from build123d import *

# Parameters (mm, degrees)
SKETCH_1_W          = 54
SKETCH_1_H          = 54
EXTRUDE_1_DEPTH     = 24
FILLET_1_R          = 2
FILLET_2_R          = 2
FILLET_3_R          = 2
FILLET_4_R          = 2
CUT_EXTRUDE_1_DEPTH = 20
SKETCH_9_R          = 2.5
SKETCH_9_R_2        = 0.75
EXTRUDE_4_DEPTH     = 6.4


with BuildPart() as part:
    # Sketch 1 → Extrude 1 (new body)
    with BuildSketch(Plane(origin=(0, 0, 0), x_dir=(1, 0, 0), z_dir=(0, 1, 0))):
        Rectangle(SKETCH_1_W, SKETCH_1_H)
    extrude(amount=EXTRUDE_1_DEPTH)

    # Fillet 1
    fillet_1_edges = [part.edges().sort_by_distance(p)[0] for p in [
        (-27, 12, 27),
    ]]
    fillet(fillet_1_edges, radius=FILLET_1_R)

    # Fillet 2
    fillet_2_edges = [part.edges().sort_by_distance(p)[0] for p in [
        (-27, 12, -27),
    ]]
    fillet(fillet_2_edges, radius=FILLET_2_R)

    # Fillet 3
    fillet_3_edges = [part.edges().sort_by_distance(p)[0] for p in [
        (27, 12, 27),
    ]]
    fillet(fillet_3_edges, radius=FILLET_3_R)

    # Fillet 4
    fillet_4_edges = [part.edges().sort_by_distance(p)[0] for p in [
        (27, 12, -27),
    ]]
    fillet(fillet_4_edges, radius=FILLET_4_R)

    # Sketch 6 → Cut-Extrude 1 (cut)
    with BuildSketch(Plane.XZ):
        with BuildLine():
            Line((-25.5, 25), (-25.5, -25))
            ThreePointArc((-25.5, -25), (-25.353553391, -25.353553391), (-25, -25.5))
            Line((-25, -25.5), (25, -25.5))
            ThreePointArc((25, -25.5), (25.353553391, -25.353553391), (25.5, -25))
            Line((25.5, -25), (25.5, 25))
            ThreePointArc((25.5, 25), (25.353553391, 25.353553391), (25, 25.5))
            Line((25, 25.5), (-25, 25.5))
            ThreePointArc((-25, 25.5), (-25.353553391, 25.353553391), (-25.5, 25))
        make_face()
    extrude(amount=-CUT_EXTRUDE_1_DEPTH, mode=Mode.SUBTRACT)

    # Sketch 9 → Extrude 4 (add)
    # profile 1 of 4: a face of its own
    with BuildSketch(Plane.XZ.offset(-20)):
        with Locations(Location((22.15, -22.5, 0), (0, 0, 270))):
            Circle(SKETCH_9_R)
        with Locations(Location((22.15, -22.5, 0), (0, 0, 270))):
            Circle(SKETCH_9_R_2, mode=Mode.SUBTRACT)
    # profile 2 of 4: a face of its own
    with BuildSketch(Plane.XZ.offset(-20)):
        with Locations(Location((-22.15, -22.5, 0), (0, 0, 270))):
            Circle(SKETCH_9_R)
        with Locations(Location((-22.15, -22.5, 0), (0, 0, 270))):
            Circle(SKETCH_9_R_2, mode=Mode.SUBTRACT)
    # profile 3 of 4: a face of its own
    with BuildSketch(Plane.XZ.offset(-20)):
        with Locations(Location((22.15, 11.8, 0), (0, 0, 270))):
            Circle(SKETCH_9_R)
        with Locations(Location((22.15, 11.8, 0), (0, 0, 270))):
            Circle(SKETCH_9_R_2, mode=Mode.SUBTRACT)
    # profile 4 of 4: a face of its own
    with BuildSketch(Plane.XZ.offset(-20)):
        with Locations(Location((-22.15, 11.8, 0), (0, 0, 270))):
            Circle(SKETCH_9_R)
        with Locations(Location((-22.15, 11.8, 0), (0, 0, 270))):
            Circle(SKETCH_9_R_2, mode=Mode.SUBTRACT)
    extrude(amount=EXTRUDE_4_DEPTH)


solid = part.part
Build history of the part. All positions in model axes, mm. A direction names the side the tool comes from. Round coordinates to 2 decimals unless told otherwise and drop trailing zeros. Loops run counter-clockwise (first coordinate to the right, second up) from the corner with the lowest first, then second, coordinate; pieces in that order, holes last. Notation, with made-up numbers: (-17, 27) -> (-2, 27) arc R29 cw to (-2, 59) -> close; hole circle Ø3 at (10, 55). An arc over 180 degrees is marked (long way). Answer in a Markdown table with one row per item.
Item 1: Pin check, flat tips, straight feed: pin 1 (0.8 mm diameter, centred on x = -22.5, z = -23, fed in from -Y); pin 2 (8 mm diameter, centred on x = -11, z = -0.5, fed in from -Y). Stop position of each tip, or through.
Answers below:
| item | result |
|---|---|
| pin 1 | stops at y = 13.6 |
| pin 2 | stops at y = 20 |
Item 2: Saw through at D-D (x = -15.5). Write the cut outline in (y, z), and give its area (3 significant figures).
Answers below:
| item | result |
|---|---|
| outline | (0, -27) -> (24, -27) -> (24, 27) -> (0, 27) -> (0, 25.5) -> (20, 25.5) -> (20, -25.5) -> (0, -25.5) -> close |
| area | 276 mm² |
Item 3: Which spindle directions (+Z, -Z, +X, -X, +Y, -Y) get a long thin tool onto all of the face, cutting with end or side? Do faces 4 (the cylindrical face through (22.18, 16.84, -21.75)), 5 (the flat face through (-2, 0, 26)). Say none if no direction does.
Answers below:
| item | result |
|---|---|
| face 4 | -Y |
| face 5 | +Z, -Z, +X, -X, -Y |
Item 4: Saw through at B-B (z = -22.5). Write the cut outline in (x, y), and give its area (3 significant figures).
Answers below:
| item | result |
|---|---|
| outline | (-27, 0) -> (-25.5, 0) -> (-25.5, 20) -> (-24.65, 20) -> (-24.65, 13.6) -> (-22.9, 13.6) -> (-22.9, 20) -> (-21.4, 20) -> (-21.4, 13.6) -> (-19.65, 13.6) -> (-19.65, 20) -> (19.65, 20) -> (19.65, 13.6) -> (21.4, 13.6) -> (21.4, 20) -> (22.9, 20) -> (22.9, 13.6) -> (24.65, 13.6) -> (24.65, 20) -> (25.5, 20) -> (25.5, 0) -> (27, 0) -> (27, 24) -> (-27, 24) -> close |
| area | 321 mm² |
Item 5: Saw through at C-C (y = 5.5). Write the cut outline in (x, z).
Answers below:
| item | result |
|---|---|
| outline | (-27, -25) arc R2 ccw to (-25, -27) -> (25, -27) arc R2 ccw to (27, -25) -> (27, 25) arc R2 ccw to (25, 27) -> (-25, 27) arc R2 ccw to (-27, 25) -> close; hole (-25.5, -25) arc R0.5 ccw to (-25, -25.5) -> (25, -25.5) arc R0.5 ccw to (25.5, -25) -> (25.5, 25) arc R0.5 ccw to (25, 25.5) -> (-25, 25.5) arc R0.5 ccw to (-25.5, 25) -> close |
Item 6: Mould opens along X. For faces 1 (the cylindrical face through (26.4, 12.17, 26.43)), 2 (the flat face through (-22, 20, -22)), 3 (the flat face through (0, 24, 0)) say: +X half, -X half, draft (parallel to the pull), parting line (faces both ways), or undercut.
Answers below:
| item | result |
|---|---|
| face 1 | +X half |
| face 2 | undercut |
| face 3 | draft |
Item 7: Drill centre lines: L1, parallel to X at y = 15.75, z = -22.5; L2, parallel to Z at x = 12, y = 10. Where is each one in solid material? Low to high. Write a range as [from, to].
Answers below:
| item | result |
|---|---|
| L1 | x = [-27, -25.5], [-24.65, -22.9], [-21.4, -19.65], [19.65, 21.4], [22.9, 24.65], [25.5, 27] |
| L2 | z = [-27, -25.5], [25.5, 27] |
Item 8: Saw through at A-A (y = 19). State how many separate pieces and enclosed holes the cut face has, and give its area (3 significant figures).
Answers below:
| item | result |
|---|---|
| separate pieces | 5 |
| enclosed holes | 5 |
| area | 383 mm² |
